Here's how the part is built. I have some questions about the finished solid (model axes, mm). A direction names the side the tool comes from. Give positions to 0.01 mm unless a question says otherwise; leave off trailing zeros. Loops run counter-clockwise (first coordinate to the right, second up) from the corner with the lowest first, then second, coordinate; pieces in that order, holes last. Notation, with made-up numbers: M 3,-14 L 26,-14 A19 cw 26,18 Z; hole C -27.75,60.25 d6. An arc over 180 degrees is marked long. Write item = value, one per line. Start each with the question number.
```python
from build123d import *

# Parameters (mm, degrees)
F1_DEPTH = 32.5
F3_DEPTH = 2.5
F4_DEPTH = 25
F5_R     = 2.5
F6_R     = 1.25


with BuildPart() as f1:
    # F0 (on Front) → F1 (new body)
    with BuildSketch(Plane.XZ):
        Polygon((-57.07207, 38.769209), (-60.82207, 38.769209), (-60.82207, 12.519209), (17.92793, 12.519209), (17.92793, 20.019209), (-25.82207, 20.019209), (-25.82207, 38.769209), (-29.57207, 38.769209), (-40.82207, 27.519209), (-40.82207, 25.019209), (-45.82207, 25.019209), (-45.82207, 27.519209), align=None)
    extrude(amount=F1_DEPTH)

    # F2 (on face) → F3 (join)
    with BuildSketch(Plane.XY.offset(20.019209)):
        with BuildLine():
            Line((4.214367, -8.75), (-13.285633, -8.75))
            ThreePointArc((-13.285633, -8.75), (-20.785633, -16.25), (-13.285633, -23.75))
            Line((-13.285633, -23.75), (4.214367, -23.75))
            ThreePointArc((4.214367, -23.75), (11.714367, -16.25), (4.214367, -8.75))
        make_face()
        with BuildLine():
            ThreePointArc((-13.285633, -20), (-17.035633, -16.25), (-13.285633, -12.5))
            Line((-13.285633, -12.5), (4.214367, -12.5))
            ThreePointArc((4.214367, -12.5), (7.964367, -16.25), (4.214367, -20))
            Line((4.214367, -20), (-13.285633, -20))
        make_face(mode=Mode.SUBTRACT)
    extrude(amount=F3_DEPTH)

    # F3_face (on face) → F4 (cut)
    with BuildSketch(Plane(origin=(-4.535633, -16.25, 20.019209), x_dir=(1, 0, 0), z_dir=(0, 0, 1))):
        with BuildLine():
            Line((8.75, 3.75), (-8.75, 3.75))
            ThreePointArc((-8.75, 3.75), (-12.5, 0), (-8.75, -3.75))
            Line((-8.75, -3.75), (8.75, -3.75))
            ThreePointArc((8.75, -3.75), (12.5, 0), (8.75, 3.75))
        make_face()
    extrude(amount=-F4_DEPTH, mode=Mode.SUBTRACT)

    # F5
    f5_edges = [f1.edges().sort_by_distance(p)[0] for p in [
        (-25.82207, -16.25, 20.019209),
    ]]
    fillet(f5_edges, radius=F5_R)

    # F6
    f6_edges = [f1.edges().sort_by_distance(p)[0] for p in [
        (-4.535633, -23.75, 20.019209),
    ]]
    fillet(f6_edges, radius=F6_R)


solid = f1.part
```
Q1. We'd pull the mould along Y, two halves only. Please class faces 1 (the flat face through (-28, -16, 38.769)), 2 (the cylindrical face through (7.963, -16.332, 17.589)), 3 (the flat face through (-31, 0, 23)): pulls with the +Y half, pulls with the -Y half, needs draft (parallel to the pull), parting line crosses it, or undercut.
Q2. If I drill on line 1 along X through (y, z) = (-15.5, 20.75); line 2 along Z through (x, y) = (-8, -26); line 3 along X through (y, z) = (-14.5, 16), over which ranges is the centre line in solid material (lowest first)?
Q3. If we section it at B-B, the plane y = -16.25: List the corners of the cut face in (x, z) for me.
Q4. Will these pins go through, and if not, where does the flat tip stop? pin 1 (16 mm diameter, centred on x = -11.5, y = -18.5, fed in from +Z); pin 2 (8 mm diameter, centred on y = -22.5, z = 32, fed in from +X); pin 3 (2.5 mm diameter, centred on x = -44.5, y = -24, fed in from +Z); pin 4 (3 mm diameter, centred on x = -23, z = 28, fed in from +Y).
Q5. If we section it at C-C, the plane x = -3: List the corners of the cut face in (y, z) for me.
Q6. If we section it at A-A, the plane z = 15.25: List the corners of the cut face in (x, y) for me.
Q7. If we section it at D-D, the plane z = 26.5: List the corners of the cut face in (x, y) for me.
Q8. On a 3-axis mill with a long thin cutter (end or side, diameter ignored), from which of +Z, -Z, +X, -X, +Y, -Y can I reach the whole of each face in a straight line? I mean faces 4 (the cylindrical face through (11.713, -16.415, 21.885)), 5 (the flat face through (-45.822, -16, 26)), 6 (the flat face through (-5, -20, 18)), 7 (the flat face through (-31, -32.5, 23)), 8 (the cylindrical face through (-20.784, -16.085, 21.885)). Say none if no direction works.
Resolved:
q1.face_1 = needs draft
q1.face_2 = undercut
q1.face_3 = pulls with the +Y half
q2.line_1 = -60.82 to -25.09, -20.86 to -16.96, 7.89 to 11.79
q2.line_2 = 12.52 to 20.02
q2.line_3 = -60.82 to -16.6, 7.53 to 17.93
q3.outline = M -60.82,12.52 L -17.04,12.52 L -17.04,22.52 L -20.79,22.52 L -20.79,21.27 A1.25 cw -22.04,20.02 L -23.32,20.02 A2.5 cw -25.82,22.52 L -25.82,38.77 L -29.57,38.77 L -40.82,27.52 L -40.82,25.02 L -45.82,25.02 L -45.82,27.52 L -57.07,38.77 L -60.82,38.77 Z; M 7.96,12.52 L 17.93,12.52 L 17.93,20.02 L 12.96,20.02 A1.25 cw 11.71,21.27 L 11.71,22.52 L 7.96,22.52 Z
q4.pin_1 = 22.52
q4.pin_2 = -25.82
q4.pin_3 = 25.02
q4.pin_4 = through
q5.outline = M -32.5,12.52 L -20,12.52 L -20,22.52 L -23.75,22.52 L -23.75,21.27 A1.25 cw -25,20.02 L -32.5,20.02 Z; M -12.5,12.52 L 0,12.52 L 0,20.02 L -7.5,20.02 A1.25 cw -8.75,21.27 L -8.75,22.52 L -12.5,22.52 Z
q6.outline = M -60.82,-32.5 L 17.93,-32.5 L 17.93,0 L -60.82,0 Z; hole M -13.29,-20 L 4.21,-20 A3.75 ccw 4.21,-12.5 L -13.29,-12.5 A3.75 ccw Z
q7.outline = M -60.82,-32.5 L -45.82,-32.5 L -45.82,0 L -60.82,0 Z; M -40.82,-32.5 L -25.82,-32.5 L -25.82,0 L -40.82,0 Z
q8.face_4 = +Z, +X
q8.face_5 = +Z, +Y, -Y
q8.face_6 = +Z, -Z
q8.face_7 = +Z, -Z, +X, -X, -Y
q8.face_8 = +Z
